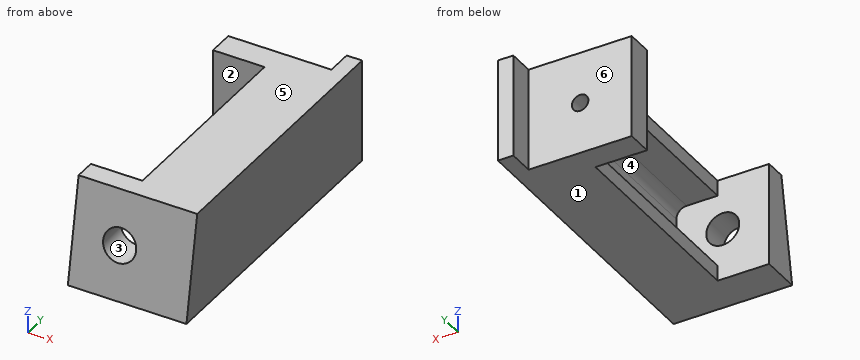
from build123d import *

# Parameters (mm, degrees)
BOSS_EXTRUDE1_DEPTH = 20
SKETCH3_R           = 1.6
CUT_EXTRUDE1_DEPTH  = 20
BOSS_EXTRUDE2_DEPTH = 40
FILLET1_R           = 2
BOSS_EXTRUDE3_DEPTH = 23
SKETCH6_R           = 3.2
CUT_EXTRUDE2_DEPTH  = 13


with BuildPart() as part:
    # Sketch2 → Boss-Extrude1 (new body)
    with BuildSketch(Plane.XY):
        Polygon((-10, 2.5), (10, 2.5), (10, 7.5), (13, 7.5), (13, -2.5), (10, -2.5), (-10, -2.5), align=None)
    extrude(amount=BOSS_EXTRUDE1_DEPTH)

    # Sketch3 → Cut-Extrude1 (cut)
    with BuildSketch(Plane(origin=(0, 2.5, 0), x_dir=(1, 0, 0), z_dir=(0, 1, 0))):
        with Locations(Location((0, -10, 0), (0, 0, 270))):
            Circle(SKETCH3_R)
    extrude(amount=-CUT_EXTRUDE1_DEPTH, mode=Mode.SUBTRACT)

    # Sketch4 → Boss-Extrude2 (add)
    with BuildSketch(Plane.XZ.offset(2.5)):
        Polygon((13, 0), (8, 0), (0, 0), (0, 3), (8, 3), (8, 17), (0, 17), (0, 20), (8, 20), (13, 20), align=None)
    extrude(amount=BOSS_EXTRUDE2_DEPTH)

    # Fillet1
    fillet1_edges = [part.edges().sort_by_distance(p)[0] for p in [
        (8, -22.5, 17),
        (8, -22.5, 3),
    ]]
    fillet(fillet1_edges, radius=FILLET1_R)

    # Sketch5 → Boss-Extrude3 (add)
    with BuildSketch(Plane(origin=(13, 0, 0), x_dir=(0, 0, -1), z_dir=(1, 0, 0))):
        Polygon((-20, -42.5), (-20, -46.5), (0, -50.026539614), (0, -42.5), align=None)
    extrude(amount=-BOSS_EXTRUDE3_DEPTH)

    # Sketch6 → Cut-Extrude2 (cut)
    with BuildSketch(Plane(origin=(0, -42.5, 0), x_dir=(1, 0, 0), z_dir=(0, 1, 0))):
        with Locations(Location((-1, -10, 0), (0, 0, 180))):
            Circle(SKETCH6_R)
    extrude(amount=-CUT_EXTRUDE2_DEPTH, mode=Mode.SUBTRACT)


solid = part.part
Can you work these out from the model? Positions are in its coordinate system, mm. Face numbers are marked on the shaded views. A direction names the side the tool comes from. Round coordinates to 2 decimals unless told otherwise and drop trailing zeros. Write each loop counter-clockwise with the first axis right and the second up, starting at its lowest first coordinate (ties: lowest second). Pieces come first, ordered by that corner, then holes. Notation, with made-up numbers: (58.25, -16) - (101.25, -16) arc R28 cw to (101.25, 6) - close; hole circle Ø7 at (51, 30.5). An arc over 180 degrees is marked (long way). Write each question's results on one line, items separated by ' | '. Start each with the question number.
1) For pin 1 Ø10 at (x, z) = (-1, 10) entering from -Y; pin 2 Ø3.5 at (x, z) = (0, 10) entering from -Y; pin 3 Ø8 at (y, z) = (-17.5, 8) entering from -X, each with a flat end and sliding along its axis, tell me the tip position at first contact or that it passes through.
2) We'd pull the mould along Z, two halves only. Please class the marked faces 4, 5 and 6: released by +Z, released by -Z, zero draft, split by the parting line, or undercut.
3) Which directions (+Z, -Z, +X, -X, +Y, -Y) give clear straight access to the entire face, cutting with the end or side of a thin tool? Please do the marked faces 1, 2 and 3.
4) Suppose I cut it at B-B (z = 10). List the corners of the cut face in (x, y) for me.
5) Please list where these lines run through material, in increasing order: line 1 (X direction, y = 0.7, z = 10); line 2 (Z direction, x = -1, y = -43.75); line 3 (X direction, y = -44, z = 10).
6) Suppose I cut it at D-D (y = -34.5). List the corners of the cut face in (x, z) for me, and give its area (3 significant figures).
7) Suppose I cut it at C-C (y = 1.5). List the corners of the cut face in (x, z) for me, and give its area (3 significant figures).
8) Suppose I cut it at A-A (x = 3.5). List the corners of the cut face in (y, z) for me, and give its area (3 significant figures).
Here are the results:
1) pin 1: stops at y = -49.14 | pin 2: stops at y = -2.5 | pin 3: stops at x = 7.73
2) face 4: undercut | face 5: released by +Z | face 6: zero draft
3) face 1: -Z, +X, -X, +Y, -Y | face 2: -X | face 3: -Y
4) outline: (-10, -48.26) - (-4.2, -48.26) - (-4.2, -42.5) - (-10, -42.5) - close; (-10, -2.5) - (-1.6, -2.5) - (-1.6, 2.5) - (-10, 2.5) - close; (1.6, -2.5) - (8, -2.5) - (8, -42.5) - (2.2, -42.5) - (2.2, -48.26) - (13, -48.26) - (13, 7.5) - (10, 7.5) - (10, 2.5) - (1.6, 2.5) - close
5) line 1: x = -10 to -1.6, 1.6 to 13 | line 2: z = 0 to 6.8, 13.2 to 20 | line 3: x = -10 to -4.2, 2.2 to 13
6) outline: (0, 0) - (13, 0) - (13, 20) - (0, 20) - (0, 17) - (6, 17) arc R2 cw to (8, 15) - (8, 5) arc R2 cw to (6, 3) - (0, 3) - close | area: 150 mm2
7) outline: (-10, 0) - (13, 0) - (13, 20) - (-10, 20) - close; hole circle Ø3.2 at (0, 10) | area: 452 mm2
8) outline: (-50.03, 0) - (2.5, 0) - (2.5, 20) - (-46.5, 20) - close; hole (-42.5, 3) - (-2.5, 3) - (-2.5, 17) - (-42.5, 17) - close | area: 455 mm2
